Part model, mm, in its own coordinate system. A direction names the side the tool comes from. Round coordinates to 2 decimals unless told otherwise and drop trailing zeros. Loops run counter-clockwise (first coordinate to the right, second up) from the corner with the lowest first, then second, coordinate; pieces in that order, holes last.
(1) Mould opens along X. For faces 1 (the face through (12, -1, 17)), 2 (the face through (-42.09, -1.52, 26.15)) say: +X half, -X half, draft (parallel to the pull), parting line (faces both ways), or undercut.
(2) Tool access for faces 3 (the face through (0, 0, 7)), 4 (the face through (-20, -2, 1.5)), 5 (the face through (37.56, -1.48, 22.75)): list every direction of +Z, -Z, +X, -X, +Y, -Y with a clear straight run to the whole face (end or side of a thin tool).
(3) Cut at B-B on z = 0. Count the separate pieces of the cut face and the enclosed holes in it, then the cut area to 3 significant figures.
(4) Flat gauge pins, fed straight in: pin 1 (8 mm diameter, centred on x = 4, y = 24.5, fed in from +Z); pin 2 (11 mm diameter, centred on x = 0, z = -4.5, fed in from +Y); pin 3 (3 mm diameter, centred on y = 35.5, z = 1.5, fed in from -X); pin 4 (6 mm diameter, centred on y = 28.5, z = -22, fed in from -X). Where does each tip first touch, or does it go through?
(5) Cut at A-A on x = 37.5. List the corners of the cut face in (y, z), then the cut area to 3 significant figures.
(6) Probe probe 1 along X at (y, z) = (-1, 0) (3 decimals); probe 2 along X at (y, z) = (8, 8.5); probe 3 along Y at (x, z) = (32, -16). List the from-to ranges inside material, lowest first.
(7) Cut at C-C on y = 26. List the corners of the cut face in (x, z), then the cut area to 3 significant figures.
from build123d import *

# Parameters (mm, degrees)
SKETCH1_W           = 86.75
SKETCH1_H           = 55
SKETCH1_R           = 5.5
BOSS_EXTRUDE1_DEPTH = 3
FILLET1_R           = 4.5
SKETCH6_R           = 19
SKETCH6_R_2         = 15.5
BOSS_EXTRUDE3_DEPTH = 45
CUT_EXTRUDE1_REACH  = 71.284
CUT_EXTRUDE1_START  = -1
CUT_EXTRUDE3_REACH  = 63.046
SKETCH12_R          = 19
SKETCH12_R_2        = 16.5
DRAFT8_ANGLE        = 2
FILLET3_R           = 2.5


with BuildPart() as part:
    # Sketch1 → Boss-Extrude1 (new body)
    with BuildSketch(Plane(origin=(0, 0, 0), x_dir=(1, 0, 0), z_dir=(0, 1, 0))):
        Rectangle(SKETCH1_W, SKETCH1_H)
        with Locations(Location((0, 0, 0), (0, 0, 270))):
            Circle(SKETCH1_R, mode=Mode.SUBTRACT)
        with BuildLine():
            Line((-34.75, 20), (-34.75, -20))
            ThreePointArc((-34.75, -20), (-37.5, -22.75), (-40.25, -20))
            Line((-40.25, -20), (-40.25, 20))
            ThreePointArc((-40.25, 20), (-37.5, 22.75), (-34.75, 20))
        make_face(mode=Mode.SUBTRACT)
        with BuildLine():
            Line((40.25, 20), (40.25, -20))
            ThreePointArc((40.25, -20), (37.5, -22.75), (34.75, -20))
            Line((34.75, -20), (34.75, 20))
            ThreePointArc((34.75, 20), (37.5, 22.75), (40.25, 20))
        make_face(mode=Mode.SUBTRACT)
    extrude(amount=-BOSS_EXTRUDE1_DEPTH)

    # Fillet1
    fillet1_edges = [part.edges().sort_by_distance(p)[0] for p in [
        (-43.375, -1.5, -27.5),
        (43.375, -1.5, -27.5),
        (43.375, -1.5, 27.5),
        (-43.375, -1.5, 27.5),
    ]]
    fillet(fillet1_edges, radius=FILLET1_R)

    # Sketch6 → Boss-Extrude3 (add)
    with BuildSketch(Plane(origin=(0, 0, 0), x_dir=(1, 0, 0), z_dir=(0, 1, 0))):
        with Locations(Location((0, 0, 0), (0, 0, 90))):
            Circle(SKETCH6_R)
        with Locations(Location((0, 0, 0), (0, 0, 90))):
            Circle(SKETCH6_R_2, mode=Mode.SUBTRACT)
    extrude(amount=BOSS_EXTRUDE3_DEPTH)

    # Sketch9 → Cut-Extrude1 (cut, up to next)
    with BuildSketch(Plane(origin=(0, 0, 0), x_dir=(1, 0, 0), z_dir=(0, 1, 0)).offset(CUT_EXTRUDE1_START), mode=Mode.PRIVATE) as cut_extrude1_sk1:
        with BuildLine():
            Line((-31.75, -22.38), (-31.75, -1.5))
            Line((-31.75, -1.5), (-7.858116823, -1.5))
            ThreePointArc((-7.858116823, -1.5), (-7.587302584, -2.536304301), (-7.180478008, -3.527142694))
            Line((-7.180478008, -3.527142694), (-31.75, -22.38))
        make_face()
    cut_extrude1_tool1 = extrude(cut_extrude1_sk1.sketch, amount=-CUT_EXTRUDE1_REACH, mode=Mode.PRIVATE) & part.part
    # Sketch9 → Cut-Extrude1 (cut, up to next)
    with BuildSketch(Plane(origin=(0, 0, 0), x_dir=(1, 0, 0), z_dir=(0, 1, 0)).offset(CUT_EXTRUDE1_START), mode=Mode.PRIVATE) as cut_extrude1_sk2:
        with BuildLine():
            Line((-31.75, 22.38), (-7.180478008, 3.527142694))
            ThreePointArc((-7.180478008, 3.527142694), (-7.587302584, 2.536304301), (-7.858116823, 1.5))
            Line((-7.858116823, 1.5), (-31.75, 1.5))
            Line((-31.75, 1.5), (-31.75, 22.38))
        make_face()
    cut_extrude1_tool2 = extrude(cut_extrude1_sk2.sketch, amount=-CUT_EXTRUDE1_REACH, mode=Mode.PRIVATE) & part.part
    # Sketch9 → Cut-Extrude1 (cut, up to next)
    with BuildSketch(Plane(origin=(0, 0, 0), x_dir=(1, 0, 0), z_dir=(0, 1, 0)).offset(CUT_EXTRUDE1_START), mode=Mode.PRIVATE) as cut_extrude1_sk3:
        with BuildLine():
            Line((-29.63, -24.5), (-1.5, -24.5))
            Line((-1.5, -24.5), (-1.5, -7.858116823))
            ThreePointArc((-1.5, -7.858116823), (-3.584038711, -7.152249053), (-5.39695236, -5.905328545))
            Line((-5.39695236, -5.905328545), (-29.63, -24.5))
        make_face()
    cut_extrude1_tool3 = extrude(cut_extrude1_sk3.sketch, amount=-CUT_EXTRUDE1_REACH, mode=Mode.PRIVATE) & part.part
    # Sketch9 → Cut-Extrude1 (cut, up to next)
    with BuildSketch(Plane(origin=(0, 0, 0), x_dir=(1, 0, 0), z_dir=(0, 1, 0)).offset(CUT_EXTRUDE1_START), mode=Mode.PRIVATE) as cut_extrude1_sk4:
        with BuildLine():
            Line((29.63, -24.5), (5.39695236, -5.905328545))
            ThreePointArc((5.39695236, -5.905328545), (3.584038711, -7.152249053), (1.5, -7.858116823))
            Line((1.5, -7.858116823), (1.5, -24.5))
            Line((1.5, -24.5), (29.63, -24.5))
        make_face()
    cut_extrude1_tool4 = extrude(cut_extrude1_sk4.sketch, amount=-CUT_EXTRUDE1_REACH, mode=Mode.PRIVATE) & part.part
    # Sketch9 → Cut-Extrude1 (cut, up to next)
    with BuildSketch(Plane(origin=(0, 0, 0), x_dir=(1, 0, 0), z_dir=(0, 1, 0)).offset(CUT_EXTRUDE1_START), mode=Mode.PRIVATE) as cut_extrude1_sk5:
        with BuildLine():
            Line((1.5, 24.5), (1.5, 7.858116823))
            ThreePointArc((1.5, 7.858116823), (3.584038711, 7.152249053), (5.39695236, 5.905328545))
            Line((5.39695236, 5.905328545), (29.63, 24.5))
            Line((29.63, 24.5), (1.5, 24.5))
        make_face()
    cut_extrude1_tool5 = extrude(cut_extrude1_sk5.sketch, amount=-CUT_EXTRUDE1_REACH, mode=Mode.PRIVATE) & part.part
    # Sketch9 → Cut-Extrude1 (cut, up to next)
    with BuildSketch(Plane(origin=(0, 0, 0), x_dir=(1, 0, 0), z_dir=(0, 1, 0)).offset(CUT_EXTRUDE1_START), mode=Mode.PRIVATE) as cut_extrude1_sk6:
        with BuildLine():
            Line((-29.63, 24.5), (-5.39695236, 5.905328545))
            ThreePointArc((-5.39695236, 5.905328545), (-3.584038711, 7.152249053), (-1.5, 7.858116823))
            Line((-1.5, 7.858116823), (-1.5, 24.5))
            Line((-1.5, 24.5), (-29.63, 24.5))
        make_face()
    cut_extrude1_tool6 = extrude(cut_extrude1_sk6.sketch, amount=-CUT_EXTRUDE1_REACH, mode=Mode.PRIVATE) & part.part
    # Sketch9 → Cut-Extrude1 (cut, up to next)
    with BuildSketch(Plane(origin=(0, 0, 0), x_dir=(1, 0, 0), z_dir=(0, 1, 0)).offset(CUT_EXTRUDE1_START), mode=Mode.PRIVATE) as cut_extrude1_sk7:
        with BuildLine():
            Line((31.75, 1.5), (31.75, 22.38))
            Line((31.75, 22.38), (7.180478008, 3.527142694))
            ThreePointArc((7.180478008, 3.527142694), (7.587302584, 2.536304301), (7.858116823, 1.5))
            Line((7.858116823, 1.5), (31.75, 1.5))
        make_face()
    cut_extrude1_tool7 = extrude(cut_extrude1_sk7.sketch, amount=-CUT_EXTRUDE1_REACH, mode=Mode.PRIVATE) & part.part
    # Sketch9 → Cut-Extrude1 (cut, up to next)
    with BuildSketch(Plane(origin=(0, 0, 0), x_dir=(1, 0, 0), z_dir=(0, 1, 0)).offset(CUT_EXTRUDE1_START), mode=Mode.PRIVATE) as cut_extrude1_sk8:
        with BuildLine():
            Line((31.75, -22.38), (7.180478008, -3.527142694))
            ThreePointArc((7.180478008, -3.527142694), (7.587302584, -2.536304301), (7.858116823, -1.5))
            Line((7.858116823, -1.5), (31.75, -1.5))
            Line((31.75, -1.5), (31.75, -22.38))
        make_face()
    cut_extrude1_tool8 = extrude(cut_extrude1_sk8.sketch, amount=-CUT_EXTRUDE1_REACH, mode=Mode.PRIVATE) & part.part
    add(cut_extrude1_tool1.solids().sort_by_distance((-22.878744, -1, 8.53751))[0], mode=Mode.SUBTRACT)
    add(cut_extrude1_tool2.solids().sort_by_distance((-22.878744, -1, -8.53751))[0], mode=Mode.SUBTRACT)
    add(cut_extrude1_tool3.solids().sort_by_distance((-11.164331, -1, 17.722088))[0], mode=Mode.SUBTRACT)
    add(cut_extrude1_tool4.solids().sort_by_distance((11.164331, -1, 17.722088))[0], mode=Mode.SUBTRACT)
    add(cut_extrude1_tool5.solids().sort_by_distance((11.164331, -1, -17.722088))[0], mode=Mode.SUBTRACT)
    add(cut_extrude1_tool6.solids().sort_by_distance((-11.164331, -1, -17.722088))[0], mode=Mode.SUBTRACT)
    add(cut_extrude1_tool7.solids().sort_by_distance((22.878744, -1, -8.53751))[0], mode=Mode.SUBTRACT)
    add(cut_extrude1_tool8.solids().sort_by_distance((22.878744, -1, 8.53751))[0], mode=Mode.SUBTRACT)

    # Sketch12 → Cut-Extrude3 (cut, up to next)
    with BuildSketch(Plane(origin=(0, 30, 0), x_dir=(1, 0, 0), z_dir=(0, 1, 0)), mode=Mode.PRIVATE) as cut_extrude3_sk1:
        with Locations(Location((0, 0, 0), (0, 0, 90))):
            Circle(SKETCH12_R)
        with Locations(Location((0, 0, 0), (0, 0, 270))):
            Circle(SKETCH12_R_2, mode=Mode.SUBTRACT)
    cut_extrude3_tool1 = extrude(cut_extrude3_sk1.sketch, amount=CUT_EXTRUDE3_REACH, mode=Mode.PRIVATE) & part.part
    add(cut_extrude3_tool1.solids().sort_by_distance((0, 30, 18.462599))[0], mode=Mode.SUBTRACT)

    # Draft8
    draft8_faces = [part.faces().sort_by_distance(p)[0] for p in [
        (0, 15, 19),
    ]]
    draft(draft8_faces, Plane.ZX, DRAFT8_ANGLE)

    # Fillet3
    fillet3_edges = [part.edges().sort_by_distance(p)[0] for p in [
        (0, 0, 19),
    ]]
    fillet(fillet3_edges, radius=FILLET3_R)


solid = part.part
Final values:
1. face 1: undercut
1. face 2: -X half
2. face 3: +Y
2. face 4: -Y
2. face 5: +Y, -Y
3. separate pieces: 4
3. enclosed holes: 0
3. area: 405 mm2
4. pin 1: stops at z = 18.21
4. pin 2: stops at y = 0
4. pin 3: stops at x = -16.5
4. pin 4: passes through
5. outline: (-3, -27.5) - (0, -27.5) - (0, -22.75) - (-3, -22.75) - close; (-3, 22.75) - (0, 22.75) - (0, 27.5) - (-3, 27.5) - close
5. area: 28.5 mm2
6. probe 1: x = -43.375 to -40.25, -34.75 to -5.5, 5.5 to 34.75, 40.25 to 43.375
6. probe 2: x = -16.68 to -12.96, 12.96 to 16.68
6. probe 3: y = -3 to 0
7. outline: circle Ø36.18 at (0, 0); hole circle Ø31 at (0, 0)
7. area: 274 mm2
